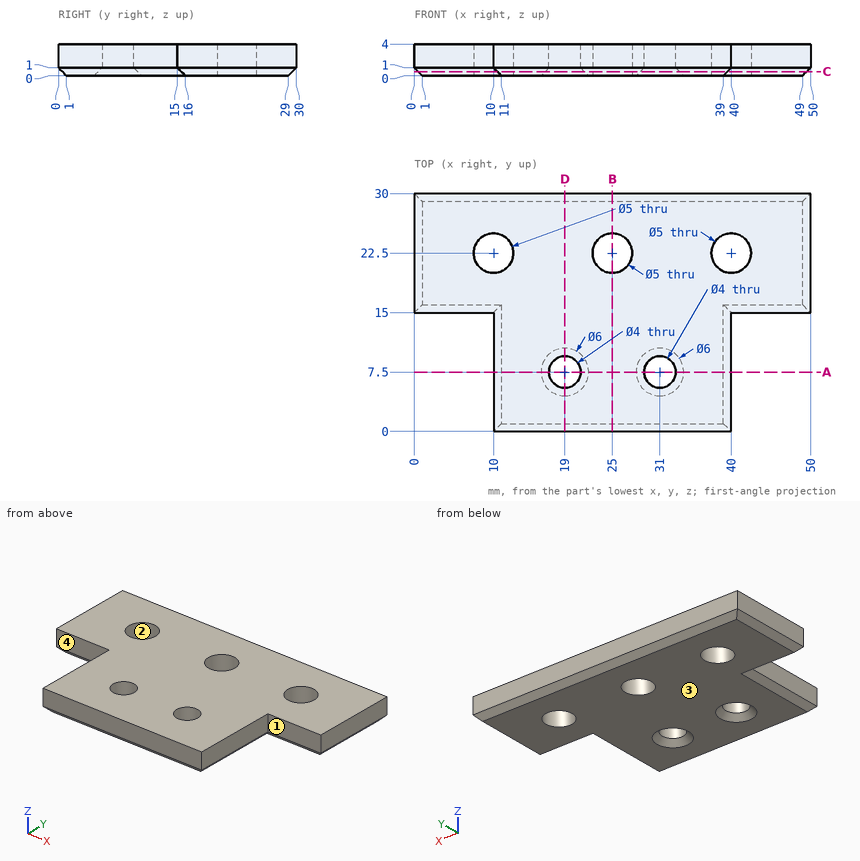
The figure shows three views and two pictorial views of one solid part (mm, origin at its lowest corner). Answer the questions. A direction names the side the tool comes from. Round coordinates to 2 decimals unless told otherwise and drop trailing zeros. Order: outer loops, then holes, each group sorted by start corner. A loop starts at its lowest first (then second) coordinate and runs counter-clockwise, first axis right, second up. Notation, with made-up numbers: (19.25, -9.5) - (30.25, -9.5) arc R26 cw to (30.25, 24.5) - close; hole circle Ø6 at (21, 83). An arc over 180 degrees is marked (long way). Write item = value, one per line. Start each with the question number.
1) Section C-C, the plane z = 0.5 is taken. Write down the section's boundary in (x, y).
2) Section B-B, the plane x = 25 is taken. Write down the section's boundary in (y, z), plus the area to 3 significant figures.
3) Given pin 1 (1.5 mm diameter, centred on y = 8.5, z = 2, fed in from -X); pin 2 (1.5 mm diameter, centred on x = 45.5, z = 2, fed in from -Y); pin 3 (3 mm diameter, centred on x = 19, y = 7.5, fed in from +Z); pin 4 (4.5 mm diameter, centred on x = 31, y = 7.5, fed in from -Z), each flat-ended and moving along its own axis, determine where each tip first touches the part or whether it passes through.
4) For a pull along X with two mould halves and no side action, classify the marked faces 1 and 2 as released by +X, released by -X, zero draft, split by the parting line, or undercut.
5) For the marked faces 3 and 4, determine the directions among +Z, -Z, +X, -X, +Y, -Y from which every point of the face is accessible in a straight line to the end or side of a thin tool.
6) Section D-D, the plane x = 19 is taken. Write down the section's boundary in (y, z), plus the area to 3 significant figures.
7) Section A-A, the plane y = 7.5 is taken. Write down the section's boundary in (x, z), plus the area to 3 significant figures.
8) Straight lines are drawn through the part: L1, parallel to X at y = 7.5, z = 2; L2, parallel to X at y = 22.5, z = 2.85; L3, parallel to X at y = 8.25, z = 2.15. For each, find the intervals that lie inside material, in ascending order.
Results list:
q1.outline = (0.5, 15.5) - (10.5, 15.5) - (10.5, 0.5) - (39.5, 0.5) - (39.5, 15.5) - (49.5, 15.5) - (49.5, 29.5) - (0.5, 29.5) - close; hole circle Ø5 at (10, 22.5); hole circle Ø5 at (19, 7.5); hole circle Ø5 at (25, 22.5); hole circle Ø5 at (31, 7.5); hole circle Ø5 at (40, 22.5)
q2.outline = (0, 1) - (1, 0) - (20, 0) - (20, 4) - (0, 4) - close; (25, 0) - (29, 0) - (30, 1) - (30, 4) - (25, 4) - close
q2.area = 99.0 mm^2
q3.pin_1 = 10
q3.pin_2 = 15
q3.pin_3 = through
q3.pin_4 = 0.75
q4.face_1 = zero draft
q4.face_2 = undercut
q5.face_3 = -Z, +X, -X, +Y, -Y
q5.face_4 = +Z, -Z, -X, -Y
q6.outline = (0, 1) - (1, 0) - (4.5, 0) - (5.5, 1) - (5.5, 4) - (0, 4) - close; (9.5, 1) - (10.5, 0) - (29, 0) - (30, 1) - (30, 4) - (9.5, 4) - close
q6.area = 102 mm^2
q7.outline = (10, 1) - (11, 0) - (16, 0) - (17, 1) - (17, 4) - (10, 4) - close; (21, 1) - (22, 0) - (28, 0) - (29, 1) - (29, 4) - (21, 4) - close; (33, 1) - (34, 0) - (39, 0) - (40, 1) - (40, 4) - (33, 4) - close
q7.area = 85.0 mm^2
q8.L1 = 10 to 17, 21 to 29, 33 to 40
q8.L2 = 0 to 7.5, 12.5 to 22.5, 27.5 to 37.5, 42.5 to 50
q8.L3 = 10 to 17.15, 20.85 to 29.15, 32.85 to 40
